from build123d import *

# Parameters (mm, degrees)
F1_W     = 45
F1_H     = 5
F1_H_2   = 6.2
F1_H_3   = 53.8
F1_R     = 1.75
F2_DEPTH = 10
F3_DEPTH = 4.22
F4_W     = 45
F4_H     = 48.8
F4_R     = 1.75
F5_DEPTH = 5


# Not quite as in the source:
# - a feature of the source that left no trace in its solid (it failed there, or was rolled back) is left out


with BuildPart() as f2:
    # F1 (on Top) → F2 (new body)
    with BuildSketch(Plane.XY):
        with Locations((0, 30)):
            Rectangle(F1_W, F1_H)
        with Locations((0, 24.4)):
            Rectangle(F1_W, F1_H_2)
        with Locations((0, -5.6)):
            Rectangle(F1_W, F1_H_3)
        with Locations((-18, -25.45)):
            Circle(F1_R, mode=Mode.SUBTRACT)
        with Locations((18, -25.45)):
            Circle(F1_R, mode=Mode.SUBTRACT)
    extrude(amount=F2_DEPTH)

    # F1 (on Top) → F3 (cut)
    with BuildSketch(Plane.XY):
        with Locations((0, 24.4)):
            Rectangle(F1_W, F1_H_2)
    extrude(amount=F3_DEPTH, mode=Mode.SUBTRACT)

    # F4 (on face) → F5 (cut)
    with BuildSketch(Plane.XY.offset(10)):
        with Locations((0, -8.1)):
            Rectangle(F4_W, F4_H)
        with Locations((-18, -25.45)):
            Circle(F4_R, mode=Mode.SUBTRACT)
        with Locations((18, -25.45)):
            Circle(F4_R, mode=Mode.SUBTRACT)
    extrude(amount=-F5_DEPTH, mode=Mode.SUBTRACT)


solid = f2.part
Geometry check sheet. Reference: the model listing, model coordinates, mm. A direction names the side the tool comes from. Round coordinates to 2 decimals unless told otherwise and drop trailing zeros. Write each loop counter-clockwise with the first axis right and the second up, starting at its lowest first coordinate (ties: lowest second). Pieces come first, ordered by that corner, then holes. Notation, with made-up numbers: (5, 29.5) - (47, 29.5) arc R26 cw to (47, 64.5) - close; hole circle Ø9 at (18.25, 1). An arc over 180 degrees is marked (long way). One line per item, written item: value.
1. Cross-section at A-A on z = 2.25. Record the boundary of the cut face in (x, y), and give its area (3 significant figures).
The answers:
outline: (-22.5, -32.5) - (22.5, -32.5) - (22.5, 21.3) - (-22.5, 21.3) - close; (-22.5, 27.5) - (22.5, 27.5) - (22.5, 32.5) - (-22.5, 32.5) - close; hole circle Ø3.5 at (-18, -25.45); hole circle Ø3.5 at (18, -25.45)
area: 2,630 mm^2
2. Scan lines: L1, parallel to Y at x = 18, z = 3.05; L2, parallel to Y at x = -17, z = 1.5; L3, parallel to X at y = -24, z = 4.75. Record each from-to range of solid material in increasing order.
The answers:
L1: y = -32.5 to -27.2, -23.7 to 21.3, 27.5 to 32.5
L2: y = -32.5 to -26.89, -24.01 to 21.3, 27.5 to 32.5
L3: x = -22.5 to -18.98, -17.02 to 17.02, 18.98 to 22.5
3. Mould release check, pull along Y, two halves, no side actions. Record for faces 4 (the face through (-19.29, -24.27, 2.46)), 5 (the face through (0, 32.5, 5)), 6 (the face through (-22.5, 0, 4)): released by +Y, released by -Y, zero draft, split by the parting line, or undercut.
The answers:
face 4: undercut
face 5: released by +Y
face 6: zero draft
4. Cross-section at D-D on x = 9.5. Record the boundary of the cut face in (y, z).
The answers:
outline: (-32.5, 0) - (21.3, 0) - (21.3, 4.22) - (27.5, 4.22) - (27.5, 0) - (32.5, 0) - (32.5, 10) - (16.3, 10) - (16.3, 5) - (-32.5, 5) - close
5. Cross-section at B-B on y = -25.45. Record the boundary of the cut face in (x, z), and give its area (3 significant figures).
The answers:
outline: (-22.5, 0) - (-19.75, 0) - (-19.75, 5) - (-22.5, 5) - close; (-16.25, 0) - (16.25, 0) - (16.25, 5) - (-16.25, 5) - close; (19.75, 0) - (22.5, 0) - (22.5, 5) - (19.75, 5) - close
area: 190 mm^2
6. Cross-section at C-C on x = 18. Record the boundary of the cut face in (y, z), and give its area (3 significant figures).
The answers:
outline: (-32.5, 0) - (-27.2, 0) - (-27.2, 5) - (-32.5, 5) - close; (-23.7, 0) - (21.3, 0) - (21.3, 4.22) - (27.5, 4.22) - (27.5, 0) - (32.5, 0) - (32.5, 10) - (16.3, 10) - (16.3, 5) - (-23.7, 5) - close
area: 362 mm^2
7. Set-up check for faces 1 (the face through (0, 25, 10)), 2 (the face through (0, 16.3, 8)), 3 (the face through (0, 27.5, 2)): record each of +Z, -Z, +X, -X, +Y, -Y from which the full face is reachable in a straight line by a thin tool's end or side.
The answers:
face 1: +Z, +X, -X, +Y, -Y
face 2: +Z, +X, -X, -Y
face 3: -Z, +X, -X
8. Depth check by flat-ended pin: pin 1 Ø3 at (x, y) = (-5.5, 23) entering from -Z; pin 2 Ø4 at (y, z) = (2.5, 7.5) entering from -X; pin 3 Ø1.5 at (x, z) = (7, 7.5) entering from -Y; pin 4 Ø1.5 at (x, y) = (6, 15.5) entering from +Z. Enter the tip coordinate at first touch or a pass-through.
The answers:
pin 1: stops at z = 4.22
pin 2: passes through
pin 3: stops at y = 16.3
pin 4: stops at z = 5
